Input: dimensioned drawing with shaded views. Units: mm. Origin: part minimum x, y, z. A direction names the side the tool comes from. Give positions to 0.01 mm unless a question says otherwise; leave off trailing zeros. Write each loop counter-clockwise with the first axis right and the second up, starting at its lowest first coordinate (ties: lowest second). Pieces come first, ordered by that corner, then holes. Notation, with made-up numbers: M 55.25,-34 L 88.25,-34 A22 cw 88.25,-13 Z; hole C -39,80.25 d2. An arc over 180 degrees is marked long. Answer as a JSON object with one key per item and string values.
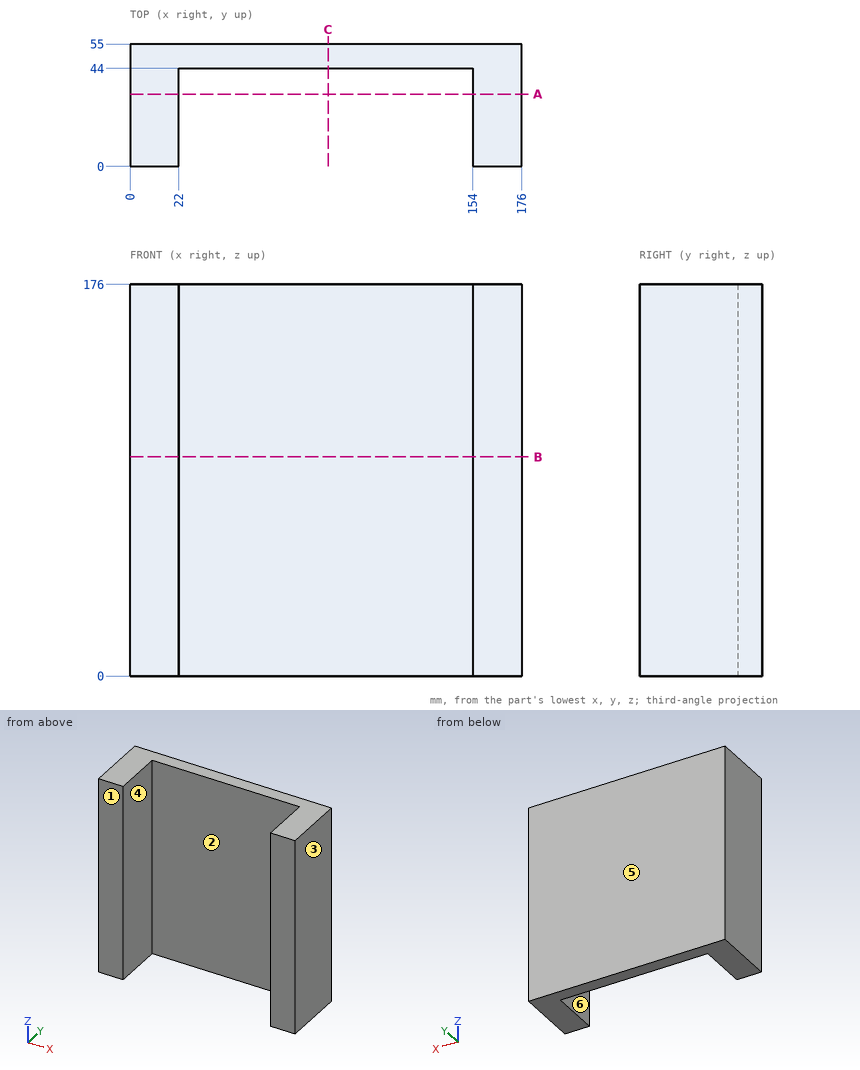
1) Cut plane A-A on y = 32.5. Return loops of the section in (x, z), and give its area (3 significant figures).
Geometry check:
{"outline": "M 0,0 L 22,0 L 22,176 L 0,176 Z; M 154,0 L 176,0 L 176,176 L 154,176 Z", "area": "7,740 mm2"}
2) Set-up query: the marked faces 5 and 6. Return all of +Z, -Z, +X, -X, +Y, -Y with unobstructed straight access to the full face (end or side cutting, diameter ignored); none if empty.
Geometry check:
{"face 5": "+Z, -Z, +X, -X, +Y", "face 6": "+Z, -Z, -Y"}
3) Pull-direction query (X, two-part tool) for the marked faces 1, 2, 3 and 4; classes: pulls with the +X half, pulls with the -X half, needs draft (parallel to the pull), parting line crosses it, or undercut.
Geometry check:
{"face 1": "needs draft", "face 2": "undercut", "face 3": "pulls with the +X half", "face 4": "undercut"}
4) Cut plane B-B on z = 98.5. Return loops of the section in (x, y).
Geometry check:
{"outline": "M 0,0 L 22,0 L 22,44 L 154,44 L 154,0 L 176,0 L 176,55 L 0,55 Z"}
5) Line query: line 1 (X direction, y = 19, z = 165); line 2 (Y direction, x = 123, z = 159). Output: solid intervals per line, ascending. Write a range as from..to.
Geometry check:
{"line 1": "x = 0..22, 154..176", "line 2": "y = 44..55"}
6) Contact query for a flat-ended pin moving along its axis: P1, Ø4, axis at x = 98.5, z = 151.5, coming from the -Y side. Output: stop coordinate, or through.
Geometry check:
{"P1": "stops at y = 44"}
7) Cut plane C-C on x = 89. Return loops of the section in (y, z), and give its area (3 significant figures).
Geometry check:
{"outline": "M 44,0 L 55,0 L 55,176 L 44,176 Z", "area": "1,940 mm2"}
